Work out the finished part from the listing and answer in its coordinate system (mm). Face numbers are marked on the shaded views. A direction names the side the tool comes from. Round coordinates to 2 decimals unless told otherwise and drop trailing zeros. Order: outer loops, then holes, each group sorted by start corner. A loop starts at its lowest first (then second) coordinate and runs counter-clockwise, first axis right, second up. Notation, with made-up numbers: (-38.5, -4) -> (-15.5, -4) arc R20 ccw to (-15.5, 24) -> close; hole circle Ø7 at (3.25, 24). An arc over 180 degrees is marked (long way). Use one line per item in the form item = value.
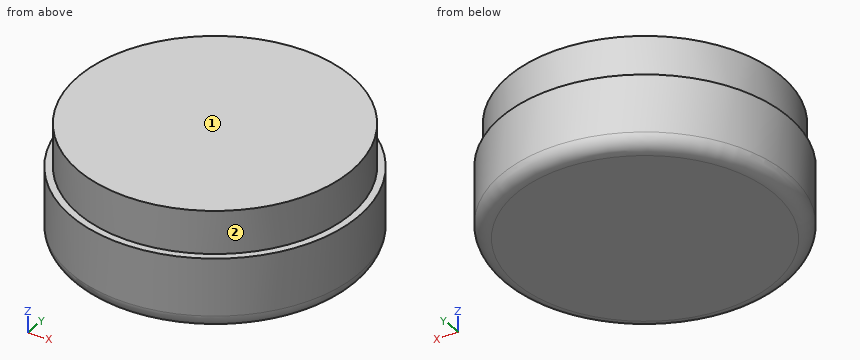
```python
from build123d import *

# Parameters (mm, degrees)
F0_R     = 9.5
F1_DEPTH = 3
F0_R_2   = 10
F2_DEPTH = 5
F3_R     = 1


with BuildPart() as f1:
    # F0 (on Top) → F1 (new body)
    with BuildSketch(Plane.XY):
        Circle(F0_R)
    extrude(amount=F1_DEPTH)

    # F0 (on Top) → F2 (join)
    with BuildSketch(Plane.XY):
        Circle(F0_R_2)
        Circle(F0_R, mode=Mode.SUBTRACT)
        Circle(F0_R)
    extrude(amount=-F2_DEPTH)

    # F3
    f3_edges = [f1.edges().sort_by_distance(p)[0] for p in [
        (-10, 0, -5),
    ]]
    fillet(f3_edges, radius=F3_R)


solid = f1.part
```
Item 1: The part is cut by section D-D, the plane z = 0.5. Give the vertices of the cut face in (x, y).
Findings:
outline = circle Ø19 at (0, 0)
Item 2: The part is cut by section C-C, the plane z = -2.25. Give the vertices of the cut face in (x, y), and give its area (3 significant figures).
Findings:
outline = circle Ø20 at (0, 0)
area = 314 mm^2
Item 3: The part is cut by section A-A, the plane x = 0. Give the vertices of the cut face in (y, z), and give its area (3 significant figures).
Findings:
outline = (-10, -4) arc R1 ccw to (-9, -5) -> (9, -5) arc R1 ccw to (10, -4) -> (10, 0) -> (9.5, 0) -> (9.5, 3) -> (-9.5, 3) -> (-9.5, 0) -> (-10, 0) -> close
area = 157 mm^2
Item 4: For the marked faces 1 and 2, determine the directions among +Z, -Z, +X, -X, +Y, -Y from which every point of the face is accessible in a straight line to the end or side of a thin tool.
Findings:
face_1 = +Z, +X, -X, +Y, -Y
face_2 = +Z
Item 5: Flat-ended cylindrical pins translate along their axes: P1, Ø1, axis at y = -1, z = -2.5, coming from the +X side; P2, Ø1.5, axis at y = 2, z = 1, coming from the -X side; P3, Ø1.5, axis at y = 5.5, z = 0.5, coming from the -X side. Find the tip coordinate at first contact, or state that the pin passes through.
Findings:
P1 = 9.99
P2 = -9.42
P3 = -8.69
Item 6: Consider line 1 along Y through (x, z) = (-7.75, -2); line 2 along X through (y, z) = (-6.25, -0.5); line 3 along Y through (x, z) = (5.75, -2.25). Determine where each line is inside the solid, lowest interval first.
Findings:
line_1 = -6.32 to 6.32
line_2 = -7.81 to 7.81
line_3 = -8.18 to 8.18
